Verification items for the finished model (mm, model axes). A direction names the side the tool comes from. Coordinates: 2 decimals unless noted, no trailing zeros. Order: outer loops, then holes, each group sorted by start corner. A loop starts at its lowest first (then second) coordinate and runs counter-clockwise, first axis right, second up. Notation, with made-up numbers: M -34.5,-16 L -26.5,-16 A13 ccw -26.5,-12 Z; hole C 69.25,4.25 d10. An arc over 180 degrees is marked long. Answer as a JSON object with one key per item and string values. Group by question number.
(1) Cross-section at C-C (x = -7). Enter the section's corners in (y, z), plus the area to 3 significant figures.
(2) Mould release check, pull along Z, two halves, no side actions. Record for faces 4 (the face through (14.94, 11, 7)), 5 (the face through (0.209, -3.117, 18.354)), 6 (the face through (0, 7, -4.02)), 7 (the face through (0.21, 10.99, 10.68)): released by +Z, released by -Z, zero draft, split by the parting line, or undercut.
(3) Cross-section at A-A (x = 0). Enter the section's corners in (y, z) (3 decimals).
(4) Access from +Z, -Z, +X, -X, +Y, -Y to the whole of each face (thin tool, end or side, straight path). Record for faces 1 (the face through (-0.209, 18.354, -3.117)), 2 (the face through (-14.94, 11, 7)), 3 (the face through (3, 0, 27)).
(5) Cross-section at B-B (y = 1). Enter the section's corners in (x, z).
(6) Gauge pin test, flat ends, axial feed: pin 1 Ø11.5 at (x, y) = (0, 31.795) entering from +Z; pin 2 Ø10 at (x, z) = (5, 30.5) entering from +Y; pin 3 Ø17 at (x, y) = (-2, 7.5) entering from +Z; pin 4 Ø4 at (x, z) = (9, 16) entering from +Y. Record the tip position at first contact, or that the pin passes through.
(7) Material ranges on line 1 (Z direction, x = 0, y = -6) (3 decimals); line 2 (Z direction, x = -9, y = 34.5), recorded low to high.
(8) Cross-section at D-D (z = 5). Enter the section's corners in (x, y), plus the area to 3 significant figures.
from build123d import *

# Parameters (mm, degrees)
BOSS_EXTRUDE1_DEPTH     = 14.94
CUT_EXTRUDE1_DEPTH      = 15.94
CUT_EXTRUDE1_DEPTH_BACK = 15.94
FILLET1_R               = 1.5
F_1_0MM_DOWEL_HOLE1_D   = 9
F_1_0MM_DOWEL_HOLE2_D   = 9
CHAMFER1_SIZE           = 0.5


with BuildPart() as part:
    # Sketch1 → Boss-Extrude1 (new body, symmetric)
    with BuildSketch(Plane(origin=(0, 0, 0), x_dir=(0, 0, -1), z_dir=(1, 0, 0))):
        Polygon((-21.67, 0), (-41.92, 0), (-41.92, -8.88), (8.88, -8.88), (8.88, 41.92), (0, 41.92), (0, 21.67), align=None)
    extrude(amount=BOSS_EXTRUDE1_DEPTH, both=True)

    # Sketch2 → Cut-Extrude1 (cut, two sides)
    with BuildSketch(Plane(origin=(0, 0, 0), x_dir=(0, 0, -1), z_dir=(1, 0, 0))) as cut_extrude1_sk:
        Polygon((-20.598831175, -4.02), (4.02, 20.598831175), (4.02, -4.02), align=None)
    extrude(amount=CUT_EXTRUDE1_DEPTH, mode=Mode.SUBTRACT)
    extrude(cut_extrude1_sk.sketch, amount=-CUT_EXTRUDE1_DEPTH_BACK, mode=Mode.SUBTRACT)

    # Fillet1
    fillet1_edges = [part.edges().sort_by_distance(p)[0] for p in [
        (0, -4.02, 20.598831175),
        (0, 20.598831175, -4.02),
    ]]
    fillet(fillet1_edges, radius=FILLET1_R)

    # Ø1.0mm Dowel Hole1 (through all)
    with Locations(Plane(origin=(0, 0, 0), x_dir=(1, 0, 0), z_dir=(0, 1, 0))):
        with Locations((0, -31.795)):
            Hole(F_1_0MM_DOWEL_HOLE1_D / 2)

    # Ø1.0mm Dowel Hole2 (through all)
    with Locations(Plane.XY):
        with Locations((0, 31.795)):
            Hole(F_1_0MM_DOWEL_HOLE2_D / 2)

    # Chamfer1
    chamfer1_edges = [part.edges().sort_by_distance(p)[0] for p in [
        (0, 0, 41.92),
        (0, 41.92, 0),
        (14.94, 31.795, 0),
        (14.94, 0, 31.795),
        (4.5, 0, 31.795),
        (4.5, 31.795, 0),
        (-14.94, 0, 31.795),
        (-14.94, 31.795, 0),
    ]]
    chamfer(chamfer1_edges, length=CHAMFER1_SIZE)


solid = part.part
Taken from the geometry:
{
 "1": {"outline": "M -8.88,-8.88 L 41.92,-8.88 L 41.92,-0.5 L 41.42,0 L 21.67,0 L 0,21.67 L 0,41.42 L -0.5,41.92 L -8.88,41.92 Z; hole M -4.02,-4.02 L 16.98,-4.02 A1.5 ccw 18.04,-1.46 L -1.46,18.04 A1.5 ccw -4.02,16.98 Z", "area": "760 mm²"},
 "2": {"face 4": "zero draft", "face 5": "undercut", "face 6": "undercut", "face 7": "released by +Z"},
 "3": {"outline": "M -8.88,-8.88 L 27.295,-8.88 L 27.295,-0.5 L 26.795,0 L 21.67,0 L 0,21.67 L 0,26.795 L -0.5,27.295 L -8.88,27.295 Z; M -8.88,36.295 L -0.5,36.295 L 0,36.795 L 0,41.42 L -0.5,41.92 L -8.88,41.92 Z; M 36.295,-8.88 L 41.92,-8.88 L 41.92,-0.5 L 41.42,0 L 36.795,0 L 36.295,-0.5 Z; hole M -4.02,-4.02 L 16.978,-4.02 A1.5 ccw 18.038,-1.459 L -1.459,18.038 A1.5 ccw -4.02,16.978 Z"},
 "4": {"face 1": "+X, -X", "face 2": "+Z, -Z, -X, +Y, -Y", "face 3": "+Z, +X, -X, +Y"},
 "5": {"outline": "M -14.94,-8.88 L 14.94,-8.88 L 14.94,-4.02 L -14.94,-4.02 Z; M -14.94,15.58 L 14.94,15.58 L 14.94,20.67 L -14.94,20.67 Z"},
 "6": {"pin 1": "stops at z = 0", "pin 2": "stops at y = 0", "pin 3": "stops at z = 41.92", "pin 4": "stops at y = 7.67"},
 "7": {"line 1": "z = -8.88 to 27.295, 36.295 to 41.92", "line 2": "z = -8.88 to 0"},
 "8": {"outline": "M -14.94,-8.88 L 14.94,-8.88 L 14.94,-4.02 L -14.94,-4.02 Z; M -14.94,11.58 L 14.94,11.58 L 14.94,16.67 L -14.94,16.67 Z", "area": "297 mm²"}
}
